```python
from build123d import *

# Parameters (mm, degrees)
ESBO_O1_W                = 60
ESBO_O1_H                = 40
RESSALTO_EXTRUS_O1_DEPTH = 20
ESBO_O8_W                = 20
ESBO_O8_H                = 20
CORTE_EXTRUS_O2_DEPTH    = 40
ESBO_O9_W                = 60
ESBO_O9_H                = 50
RESSALTO_EXTRUS_O2_DEPTH = 20


with BuildPart() as part:
    # Esboço1 → Ressalto-extrusão1 (new body)
    with BuildSketch(Plane.XY):
        with Locations((30, 20)):
            Rectangle(ESBO_O1_W, ESBO_O1_H)
    extrude(amount=RESSALTO_EXTRUS_O1_DEPTH)

    # Esboço8 → Corte-extrusão2 (cut)
    with BuildSketch(Plane.XY.offset(20)):
        with Locations((30, 10)):
            Rectangle(ESBO_O8_W, ESBO_O8_H)
    extrude(amount=-CORTE_EXTRUS_O2_DEPTH, mode=Mode.SUBTRACT)

    # Esboço9 → Ressalto-extrusão2 (add)
    with BuildSketch(Plane(origin=(0, 40, 0), x_dir=(1, 0, 0), z_dir=(0, 1, 0))):
        with Locations((30, -25)):
            Rectangle(ESBO_O9_W, ESBO_O9_H)
    extrude(amount=RESSALTO_EXTRUS_O2_DEPTH)


solid = part.part
```
Check sheet for the modelled part. Datum: model origin and axes. Units: mm. A direction names the side the tool comes from. Give positions to 0.01 mm unless a question says otherwise; leave off trailing zeros. Write each loop counter-clockwise with the first axis right and the second up, starting at its lowest first coordinate (ties: lowest second). Pieces come first, ordered by that corner, then holes.
Item 1: Cross-section at A-A (y = 15). Enter the section's corners in (x, z), and give its area (3 significant figures).
Item 2: Cross-section at B-B (z = 18.5). Enter the section's corners in (x, y), and give its area (3 significant figures).
Item 3: Scan lines: L1, parallel to X at y = 15.5, z = 19; L2, parallel to Z at x = 43.5, y = 25; L3, parallel to Y at x = 26, z = 38. Record each from-to range of solid material in increasing order.
Item 4: Cross-section at C-C (x = 28.5). Enter the section's corners in (y, z).
Item 5: Access from +Z, -Z, +X, -X, +Y, -Y to the whole of each face (thin tool, end or side, straight path). Record for faces 1 (the face through (30, 20, 10)), 2 (the face through (30, 40, 35)), 3 (the face through (50, 0, 10)).
Item 6: Cross-section at D-D (x = 55.5). Enter the section's corners in (y, z).
Item 7: Gauge pin test, flat ends, axial feed: pin 1 (10 mm diameter, centred on x = 9.5, z = 5.5, fed in from -Y); pin 2 (24 mm diameter, centred on x = 25.5, z = 40.5, fed in from -Y); pin 3 (10 mm diameter, centred on x = 28, z = 12.5, fed in from -Y); pin 4 (12 mm diameter, centred on x = 26, y = 21.5, fed in from +Z). Record the tip position at first contact, or that the pin passes through.
Item 8: Draft check along X on faces 4 (the face through (0, 36.2, 19.8)), 5 (the face through (40, 10, 10)), 6 (the face through (20, 10, 10)), 7 (the face through (30, 50, 50)). Enter one of: released by +X, released by -X, zero draft, split by the parting line, or undercut.
Report:
1. outline: (0, 0) - (20, 0) - (20, 20) - (0, 20) - close; (40, 0) - (60, 0) - (60, 20) - (40, 20) - close
1. area: 800 mm2
2. outline: (0, 0) - (20, 0) - (20, 20) - (40, 20) - (40, 0) - (60, 0) - (60, 60) - (0, 60) - close
2. area: 3,200 mm2
3. L1: x = 0 to 20, 40 to 60
3. L2: z = 0 to 20
3. L3: y = 40 to 60
4. outline: (20, 0) - (60, 0) - (60, 50) - (40, 50) - (40, 20) - (20, 20) - close
5. face 1: +Z, -Z, -Y
5. face 2: +Z, +X, -X, -Y
5. face 3: +Z, -Z, +X, -X, -Y
6. outline: (0, 0) - (60, 0) - (60, 50) - (40, 50) - (40, 20) - (0, 20) - close
7. pin 1: stops at y = 0
7. pin 2: stops at y = 40
7. pin 3: stops at y = 20
7. pin 4: stops at z = 20
8. face 4: released by -X
8. face 5: undercut
8. face 6: undercut
8. face 7: zero draft
